Source: three-view drawing plus pictorial views. Frame: mm from the lowest corner of the part. A direction names the side the tool comes from. Give positions to 0.01 mm unless a question says otherwise; leave off trailing zeros. Order: outer loops, then holes, each group sorted by start corner. A loop starts at its lowest first (then second) coordinate and runs counter-clockwise, first axis right, second up. Notation, with made-up numbers: (76.25, 78.5) -> (106.25, 78.5) arc R33 cw to (106.25, 116.5) -> close; hole circle Ø6 at (1.25, -16). An arc over 180 degrees is marked (long way). Write item = value, one per line.
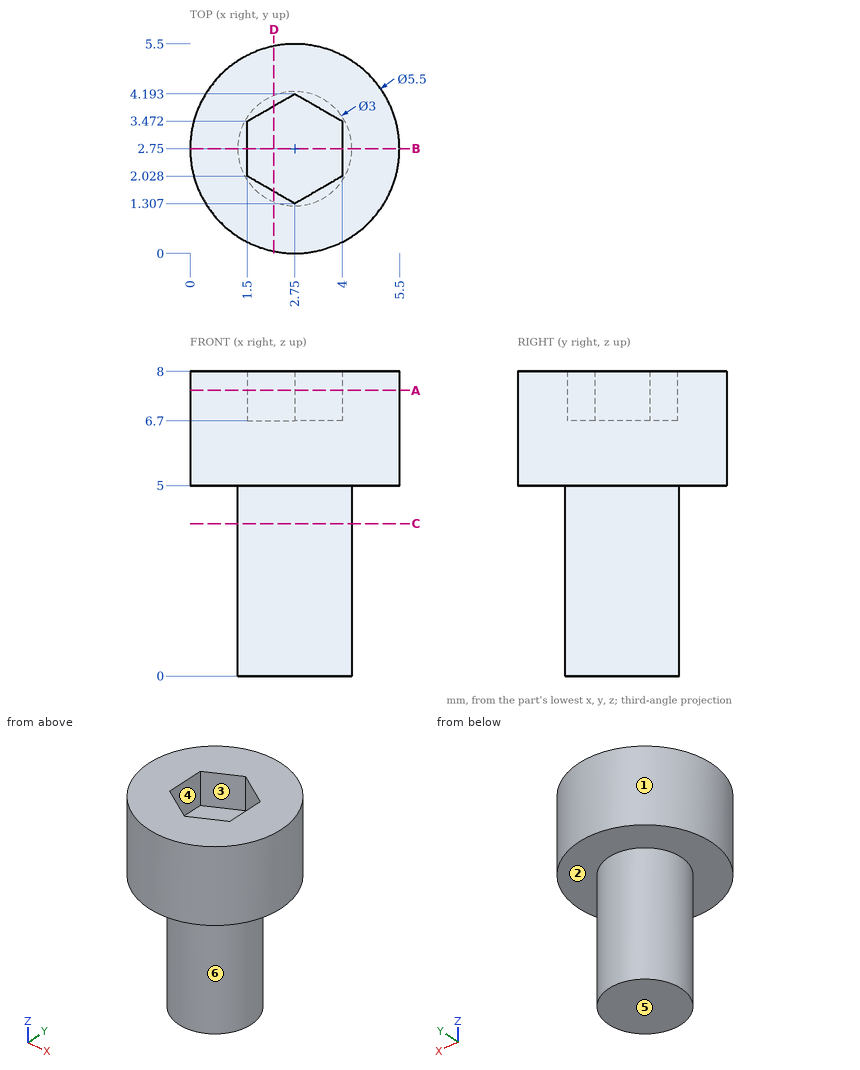
1) Section query C-C (z = 4). Output: boundary loops of the cut face in (x, y).
Check sheet entries:
outline = circle Ø3 at (2.75, 2.75)
2) Reachability of the marked faces 4, 5 and 6 from +Z, -Z, +X, -X, +Y, -Y: full face, straight path, thin tool, end or side. Return the list, or none.
Check sheet entries:
face_4 = +Z
face_5 = -Z, +X, -X, +Y, -Y
face_6 = -Z
3) Line query: line 1 (Y direction, x = 2.75, z = 3); line 2 (Z direction, x = 3, y = 3.95); line 3 (X direction, y = 2.85, z = 7.75). Output: solid intervals per line, ascending. Write a range as from..to.
Check sheet entries:
line_1 = 1.25..4.25
line_2 = 0..6.7
line_3 = 0..1.5, 4..5.5
4) Section query B-B (y = 2.75). Output: boundary loops of the cut face in (x, z).
Check sheet entries:
outline = (0, 5) -> (1.25, 5) -> (1.25, 0) -> (4.25, 0) -> (4.25, 5) -> (5.5, 5) -> (5.5, 8) -> (4, 8) -> (4, 6.7) -> (1.5, 6.7) -> (1.5, 8) -> (0, 8) -> close
5) Section query D-D (x = 2.2). Output: boundary loops of the cut face in (y, z) (1 decimal).
Check sheet entries:
outline = (0.1, 5) -> (1.4, 5) -> (1.4, 0) -> (4.1, 0) -> (4.1, 5) -> (5.4, 5) -> (5.4, 8) -> (3.9, 8) -> (3.9, 6.7) -> (1.6, 6.7) -> (1.6, 8) -> (0.1, 8) -> close
6) First-contact query: P1, Ø2, axis at x = 1, z = 2, coming from the -Y side; P2, Ø1.3, axis at x = 2.5, y = 2.5, coming from the +Z side; P3, Ø1, axis at x = 5, y = 3, coming from the -Z side. Flat tips, straight axial feed; report the tip coordinate or a pass-through.
Check sheet entries:
P1 = 1.45
P2 = 6.7
P3 = 5
7) Mould query, pull axis Y, two halves, no side actions, for the marked faces 1, 2 and 3. Classes: +Y half, -Y half, draft (parallel to the pull), parting line (faces both ways), or undercut.
Check sheet entries:
face_1 = parting line
face_2 = draft
face_3 = undercut
8) Section query A-A (z = 7.5). Output: boundary loops of the cut face in (x, y).
Check sheet entries:
outline = circle Ø5.5 at (2.75, 2.75); hole (1.5, 2.03) -> (2.75, 1.31) -> (4, 2.03) -> (4, 3.47) -> (2.75, 4.19) -> (1.5, 3.47) -> close
